Can you work these out from the drawing? Everything is in mm from the part's minimum corner. A direction names the side the tool comes from. Coordinates: 2 decimals unless noted, no trailing zeros. Loops run counter-clockwise (first coordinate to the right, second up) from the corner with the lowest first, then second, coordinate; pieces in that order, holes last.
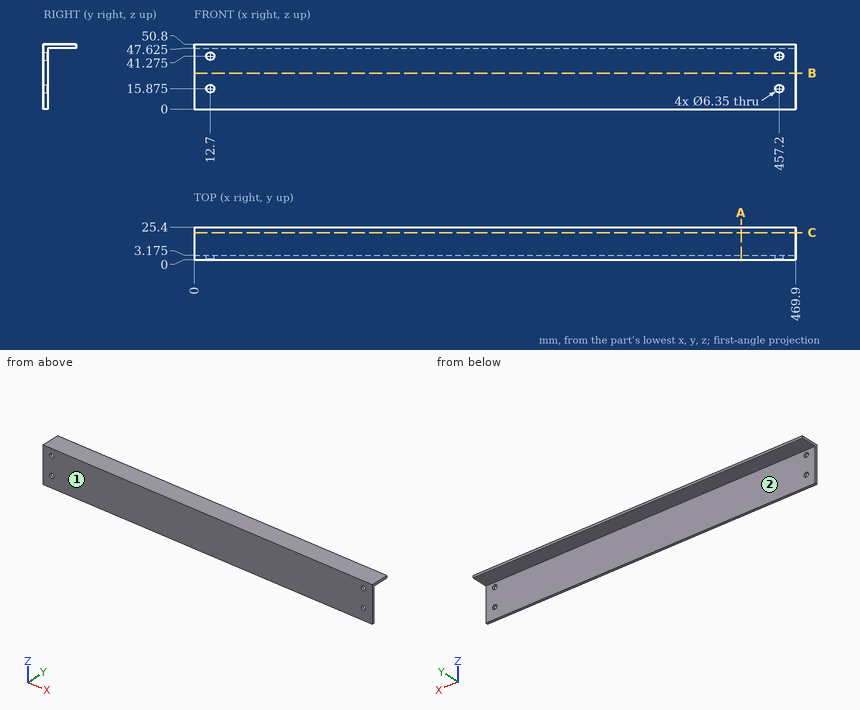
(1) For pin 1 (1.5 mm diameter, centred on x = 268, z = 13, fed in from +Y) (3 decimals); pin 2 (11 mm diameter, centred on x = 209, y = 18.5, fed in from -Z) (3 decimals), each with a flat end and sliding along its axis, tell me the tip position at first contact or that it passes through.
Answers:
pin 1: stops at y = 3.175
pin 2: stops at z = 47.625
(2) Imagine slicing it at C-C, the plane y = 21. Write out the boundary of the cut face in (x, z) (3 decimals), and give its area (3 significant figures).
Answers:
outline: (0, 47.625) - (469.9, 47.625) - (469.9, 50.8) - (0, 50.8) - close
area: 1,490 mm2
(3) I need wall thicknesses on probe 1 along Z at (x, y) = (12.7, 2.5); probe 2 along Y at (x, z) = (383.5, 7.5) (3 decimals); probe 3 along Z at (x, y) = (314, 12.5) (3 decimals). Which ranges of each line are inside material? Lowest first, please.
Answers:
probe 1: z = 0 to 12.7, 19.05 to 38.1, 44.45 to 50.8
probe 2: y = 0 to 3.175
probe 3: z = 47.625 to 50.8
(4) Which directions (+Z, -Z, +X, -X, +Y, -Y) give clear straight access to the entire face, cutting with the end or side of a thin tool? Please do the marked faces 1 and 2.
Answers:
face 1: +Z, -Z, +X, -X, -Y
face 2: -Z, +X, -X, +Y
(5) Imagine slicing it at A-A, the plane x = 427.5. Write out the boundary of the cut face in (y, z) (3 decimals).
Answers:
outline: (0, 0) - (3.175, 0) - (3.175, 47.625) - (25.4, 47.625) - (25.4, 50.8) - (0, 50.8) - close
(6) Imagine slicing it at B-B, the plane z = 28. Write out the boundary of the cut face in (x, y) (3 decimals), and give its area (3 significant figures).
Answers:
outline: (0, 0) - (469.9, 0) - (469.9, 3.175) - (0, 3.175) - close
area: 1,490 mm2
